The model under review builds one solid part; all positions refer to its coordinate system, in mm. A direction names the side the tool comes from. Round coordinates to 2 decimals unless told otherwise and drop trailing zeros. Order: outer loops, then holes, each group sorted by start corner. A loop starts at its lowest first (then second) coordinate and runs counter-clockwise, first axis right, second up.
```python
from build123d import *

# Parameters (mm, degrees)
F0_R     = 18.161
F0_R_2   = 13.3985
F1_DEPTH = 19.05
F2_R     = 21.336
F2_R_2   = 13.3985
F3_DEPTH = 6.35
F4_R     = 15.875
F4_R_2   = 11.90625
F5_DEPTH = 12.7
F6_R     = 15.875
F7_DEPTH = 19.05


with BuildPart() as f1:
    # F0 (on Front) → F1 (new body)
    with BuildSketch(Plane.XZ):
        Circle(F0_R)
        Circle(F0_R_2, mode=Mode.SUBTRACT)
    extrude(amount=F1_DEPTH)

    # F2 (on Front) → F3 (join)
    with BuildSketch(Plane.XZ):
        Circle(F2_R)
        Circle(F2_R_2, mode=Mode.SUBTRACT)
    extrude(amount=-F3_DEPTH)

    # F4 (on face) → F5 (join)
    with BuildSketch(Plane(origin=(0, 6.35, 0), x_dir=(-1, 0, 0), z_dir=(0, 1, 0))):
        Circle(F4_R)
        Circle(F4_R_2, mode=Mode.SUBTRACT)
    extrude(amount=F5_DEPTH)

    # F6 (on face) → F7 (join)
    with BuildSketch(Plane(origin=(0, 19.05, 0), x_dir=(-1, 0, 0), z_dir=(0, 1, 0))):
        Circle(F6_R)
        with BuildLine():
            ThreePointArc((-4.7625, -6.35), (-6.874077, -3.96875), (-7.880511, -0.949446))
            Line((-7.880511, -0.949446), (-11.525237, 2.987925))
            ThreePointArc((-11.525237, 2.987925), (-10.311115, 5.953125), (-8.350237, 8.487186))
            Line((-8.350237, 8.487186), (-3.118011, 7.299446))
            ThreePointArc((-3.118011, 7.299446), (0, 7.9375), (3.118011, 7.299446))
            Line((3.118011, 7.299446), (8.350237, 8.487186))
            ThreePointArc((8.350237, 8.487186), (10.311115, 5.953125), (11.525237, 2.987925))
            Line((11.525237, 2.987925), (7.880511, -0.949446))
            ThreePointArc((7.880511, -0.949446), (6.874077, -3.96875), (4.7625, -6.35))
            Line((4.7625, -6.35), (3.175, -11.475111))
            ThreePointArc((3.175, -11.475111), (0, -11.90625), (-3.175, -11.475111))
            Line((-3.175, -11.475111), (-4.7625, -6.35))
        make_face(mode=Mode.SUBTRACT)
    extrude(amount=F7_DEPTH)


solid = f1.part
```
(1) For faces 4 (the cylindrical face through (3.441, 22.003, -15.497)), 5 (the cylindrical face through (6.85, 28.44, -4.01)), 6 (the cylindrical face through (-10.633, -6.172, -8.153)), list the 3-axis set-ups (+Z, -Z, +X, -X, +Y, -Y) from which the entire face can be reached by the end or side of a thin tool; tool diameter is ignored.
Data:
face 4: +Y
face 5: +Y, -Y
face 6: -Y
(2) Draft analysis for pull direction Z (two halves, no side actions). For faces 1 (the cylindrical face through (9.845, 3.131, -18.929)), 2 (the flat face through (9, 19.05, -4)), 3 (the flat face through (-7, 38.1, -7)), state which applies: pulls with the +Z half, pulls with the -Z half, needs draft (parallel to the pull), parting line crosses it, or undercut.
Data:
face 1: parting line crosses it
face 2: undercut
face 3: needs draft
(3) Consider section C-C (y = -14). Write out the cut boundary in (x, z), and give its area (3 significant figures).
Data:
outline: circle Ø36.32 at (0, 0); hole circle Ø26.8 at (0, 0)
area: 472 mm2
(4) To check wall thickness, follow probe 1 along Z at (x, y) = (0, 15) (3 decimals); probe 2 along Z at (x, y) = (0, -5.5); probe 3 along Y at (x, z) = (1, 17). State the ranges of each line that lie inside material, in increasing order.
Data:
probe 1: z = -15.875 to -11.906, 11.906 to 15.875
probe 2: z = -18.16 to -13.4, 13.4 to 18.16
probe 3: y = -19.05 to 6.35
(5) Consider section B-B (z = -3). Write out the cut boundary in (x, y), and give its area (3 significant figures).
Data:
outline: (-21.12, 0) - (-17.91, 0) - (-17.91, -19.05) - (-13.06, -19.05) - (-13.06, 6.35) - (-11.52, 6.35) - (-11.52, 19.05) - (-7.35, 19.05) - (-7.35, 38.1) - (-15.59, 38.1) - (-15.59, 6.35) - (-21.12, 6.35) - close; (7.35, 19.05) - (11.52, 19.05) - (11.52, 6.35) - (13.06, 6.35) - (13.06, -19.05) - (17.91, -19.05) - (17.91, 0) - (21.12, 0) - (21.12, 6.35) - (15.59, 6.35) - (15.59, 38.1) - (7.35, 38.1) - close
area: 705 mm2
(6) Consider section D-D (x = 10). Write out the cut boundary in (y, z), and give its area (3 significant figures).
Data:
outline: (-19.05, -15.16) - (0, -15.16) - (0, -18.85) - (6.35, -18.85) - (6.35, -12.33) - (38.1, -12.33) - (38.1, 1.34) - (19.05, 1.34) - (19.05, -6.46) - (6.35, -6.46) - (6.35, -8.92) - (-19.05, -8.92) - close; (-19.05, 8.92) - (6.35, 8.92) - (6.35, 6.46) - (38.1, 6.46) - (38.1, 12.33) - (6.35, 12.33) - (6.35, 18.85) - (0, 18.85) - (0, 15.16) - (-19.05, 15.16) - close
area: 885 mm2
(7) Insertion check: pin 1 (8 mm diameter, centred on x = 12.5, y = 25.5, fed in from +Z); pin 2 (24 mm diameter, centred on x = 0, z = 0, fed in from -Y); pin 3 (3 mm diameter, centred on x = 8, z = -16, fed in from +Y). Each pin has a flat end and moves straight along its axis. Give the tip position at first contact, or say it passes through.
Data:
pin 1: stops at z = 13.41
pin 2: stops at y = 6.35
pin 3: stops at y = 6.35
